Input: part model. Units: mm. Frame: model coordinates. Face numbers are marked on the shaded views. A direction names the side the tool comes from. Coordinates: 2 decimals unless noted, no trailing zeros. Order: outer loops, then holes, each group sorted by start corner. A loop starts at its lowest first (then second) coordinate and runs counter-clockwise, first axis right, second up. Notation, with made-up numbers: M -15.75,47 L 2.25,47 A10 ccw 2.25,52 Z; hole C 75,37.25 d1. An arc over 180 degrees is marked long. One line per item, written item: value.
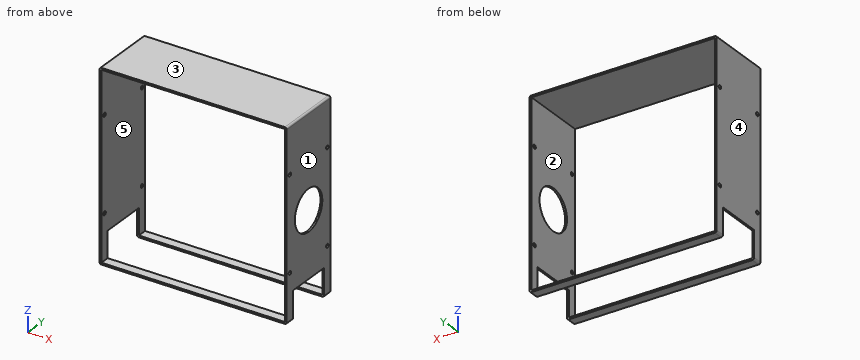
```python
from build123d import *

# Parameters (mm, degrees)
SKETCH1_W           = 100
SKETCH1_H           = 100
BOSS_EXTRUDE1_DEPTH = 35
SKETCH2_W           = 98
SKETCH2_H           = 98
CUT_EXTRUDE1_DEPTH  = 35
SKETCH5_W           = 50
SKETCH5_H           = 25
CUT_EXTRUDE2_DEPTH  = 15
SKETCH6_R           = 1
CUT_EXTRUDE4_DEPTH  = 114
SKETCH7_R           = 11
CUT_EXTRUDE5_DEPTH  = 10
FILLET1_R           = 1


with BuildPart() as part:
    # Sketch1 → Boss-Extrude1 (new body)
    with BuildSketch(Plane(origin=(0, 0, 0), x_dir=(1, 0, 0), z_dir=(0, 1, 0))):
        Rectangle(SKETCH1_W, SKETCH1_H)
    extrude(amount=BOSS_EXTRUDE1_DEPTH)

    # Sketch2 → Cut-Extrude1 (cut)
    with BuildSketch(Plane(origin=(0, 35, 0), x_dir=(1, 0, 0), z_dir=(0, 1, 0))):
        Rectangle(SKETCH2_W, SKETCH2_H)
    extrude(amount=-CUT_EXTRUDE1_DEPTH, mode=Mode.SUBTRACT)

    # Sketch5 → Cut-Extrude2 (cut)
    with BuildSketch(Plane(origin=(0, 0, -50), x_dir=(-1, 0, 0), z_dir=(0, 0, -1))):
        with Locations((-25, 17.5)):
            Rectangle(SKETCH5_W, SKETCH5_H)
        with Locations((25, 17.5)):
            Rectangle(SKETCH5_W, SKETCH5_H)
    extrude(amount=-CUT_EXTRUDE2_DEPTH, mode=Mode.SUBTRACT)

    # Sketch6 → Cut-Extrude4 (cut)
    with BuildSketch(Plane.ZY.offset(50)):
        with Locations((-25, 32.5)):
            Circle(SKETCH6_R)
        with Locations((25, 32.5)):
            Circle(SKETCH6_R)
        with Locations((-25, 2.5)):
            Circle(SKETCH6_R)
        with Locations((25, 2.5)):
            Circle(SKETCH6_R)
    extrude(amount=-CUT_EXTRUDE4_DEPTH, mode=Mode.SUBTRACT)

    # Sketch7 → Cut-Extrude5 (cut)
    with BuildSketch(Plane(origin=(50, 0, 0), x_dir=(0, 0, -1), z_dir=(1, 0, 0))):
        with Locations((0, 17.5)):
            Circle(SKETCH7_R)
    extrude(amount=-CUT_EXTRUDE5_DEPTH, mode=Mode.SUBTRACT)

    # Fillet1
    fillet1_edges = [part.edges().sort_by_distance(p)[0] for p in [
        (-50, 2.5, -50),
        (50, 2.5, -50),
        (50, 17.5, 50),
        (-50, 17.5, 50),
        (-50, 32.5, -50),
        (50, 32.5, -50),
    ]]
    fillet(fillet1_edges, radius=FILLET1_R)


solid = part.part
```
(1) Cut plane C-C on z = -6.5. Output: boundary loops of the cut face in (x, y), plus the area to 3 significant figures.
Data:
outline: M -50,0 L -49,0 L -49,35 L -50,35 Z; M 49,0 L 50,0 L 50,8.63 L 49,8.63 Z; M 49,26.37 L 50,26.37 L 50,35 L 49,35 Z
area: 52.3 mm2
(2) Ray query, line 1 (Z direction, x = 2, y = 30.5); line 2 (Z direction, x = 41.5, y = 16.5). Return the intervals inside material, ascending. Write a range as from..to.
Data:
line 1: z = -50..-49, 49..50
line 2: z = 49..50
(3) Cut plane A-A on y = 21.5. Output: boundary loops of the cut face in (x, z), plus the area to 3 significant figures.
Data:
outline: M -50,-35 L -49,-35 L -49,49 L 49,49 L 49,10.25 L 50,10.25 L 50,49 A1 ccw 49,50 L -49,50 A1 ccw -50,49 Z; M 49,-35 L 50,-35 L 50,-10.25 L 49,-10.25 Z
area: 247 mm2
(4) First-contact query: pin 1 (0.8 mm diameter, centred on x = 49.5, y = 16, fed in from -Z); pin 2 (17.5 mm diameter, centred on y = 17.5, z = 0, fed in from +X); pin 3 (1.5 mm diameter, centred on x = 3.5, y = 25, fed in from -Z). Flat tips, straight axial feed; report the tip coordinate or a pass-through.
Data:
pin 1: stops at z = -35
pin 2: stops at x = -49
pin 3: stops at z = 49
(5) Draft query along Z for the marked faces 3, 4 and 5. Return one class per face: released by +Z, released by -Z, zero draft, split by the parting line, or undercut.
Data:
face 3: released by +Z
face 4: zero draft
face 5: undercut
(6) Access query for the marked faces 1 and 2. Directions: +Z, -Z, +X, -X, +Y, -Y. A direction counts if a zero-diameter tool reaches every point of the face in a straight line with its end or side. Return the directions, or none.
Data:
face 1: +Z, -Z, +X, +Y, -Y
face 2: +Y, -Y
(7) Cut plane D-D on y = 11.5. Output: boundary loops of the cut face in (x, z).
Data:
outline: M -50,-35 L -49,-35 L -49,49 L 49,49 L 49,9.22 L 50,9.22 L 50,49 A1 ccw 49,50 L -49,50 A1 ccw -50,49 Z; M 49,-35 L 50,-35 L 50,-9.22 L 49,-9.22 Z
(8) Cut plane B-B on x = 10. Output: boundary loops of the cut face in (y, z), plus the area to 3 significant figures.
Data:
outline: M 0,-50 L 5,-50 L 5,-49 L 0,-49 Z; M 0,49 L 35,49 L 35,50 L 0,50 Z; M 30,-50 L 35,-50 L 35,-49 L 30,-49 Z
area: 45.0 mm2
